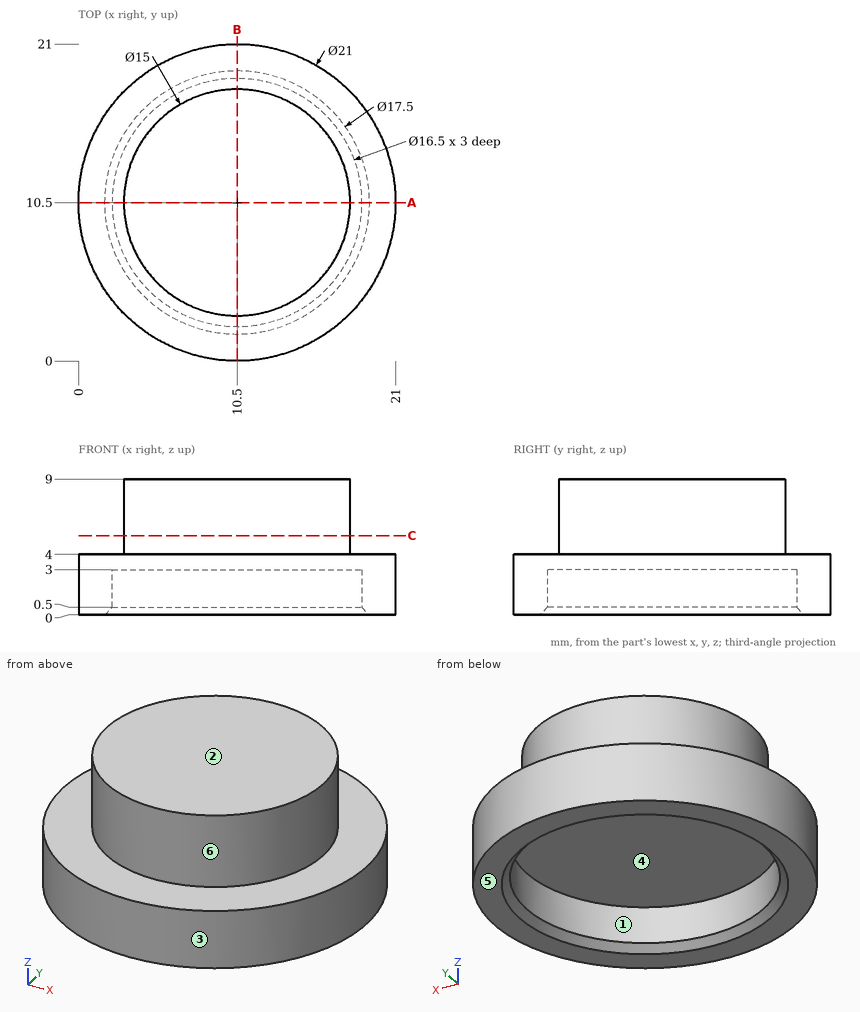
Source: three-view drawing plus pictorial views. Frame: mm from the lowest corner of the part. A direction names the side the tool comes from. Give positions to 0.01 mm unless a question says otherwise; leave off trailing zeros. Order: outer loops, then holes, each group sorted by start corner. A loop starts at its lowest first (then second) coordinate and runs counter-clockwise, first axis right, second up. Notation, with made-up numbers: M 46.25,69 L 50.25,69 A26 ccw 50.25,99 Z; hole C 48,15.5 d2. An arc over 180 degrees is marked long. One line per question, with ' | ' between items. Start each with the question number.
1. Section query A-A (y = 10.5). Return the cut outline in (x, z).
2. Access query for the marked faces 4, 5 and 6. Directions: +Z, -Z, +X, -X, +Y, -Y. A direction counts if a zero-diameter tool reaches every point of the face in a straight line with its end or side. Return the directions, or none.
3. Pull-direction query (X, two-part tool) for the marked faces 1, 2 and 3; classes: released by +X, released by -X, zero draft, split by the parting line, or undercut.
4. Section query C-C (z = 5.25). Return the cut outline in (x, y).
5. Material intervals for probe 1 along Y at (x, z) = (10.5, 1.6); probe 2 along Z at (x, y) = (11, 11.25); probe 3 along Z at (x, y) = (15.75, 1.5), sorted ascending. Write a range as [from, to].
6. First-contact query: pin 1 Ø4 at (y, z) = (14, 2.5) entering from -X; pin 2 Ø1.5 at (y, z) = (6, 7.5) entering from +X; pin 3 Ø2 at (x, z) = (7, 2.5) entering from +Y. Flat tips, straight axial feed; report the tip coordinate or a pass-through.
Here are the results:
1) outline: M 0,0 L 1.75,0 L 2.25,0.5 L 2.25,3 L 18.75,3 L 18.75,0.5 L 19.25,0 L 21,0 L 21,4 L 18,4 L 18,9 L 3,9 L 3,4 L 0,4 Z
2) face 4: -Z | face 5: -Z, +X, -X, +Y, -Y | face 6: +Z
3) face 1: undercut | face 2: zero draft | face 3: split by the parting line
4) outline: C 10.5,10.5 d15
5) probe 1: [0, 2.25], [18.75, 21] | probe 2: [3, 9] | probe 3: [0, 4]
6) pin 1: x = 0.11 | pin 2: x = 17 | pin 3: y = 20.7
